```python
from build123d import *

# Parameters (mm, degrees)
SKETCH1_R               = 3.5
BOSS_EXTRUDE1_DEPTH     = 5
BOSS_EXTRUDE2_DEPTH     = 15
CHAMFER1_SIZE           = 5
CHAMFER2_SIZE           = 5
CUT_EXTRUDE1_DEPTH      = 32.721443851
CUT_EXTRUDE1_DEPTH_BACK = 32.721443851
SKETCH3_R               = 1.5
CHAMFER3_SIZE           = 2


with BuildPart() as part:
    # Sketch1 → Boss-Extrude1 (new body)
    with BuildSketch(Plane(origin=(0, 0, 0), x_dir=(1, 0, 0), z_dir=(0, 1, 0))):
        with BuildLine():
            Line((0, 6), (15.5, 6))
            ThreePointArc((15.5, 6), (21.5, 0), (15.5, -6))
            Line((15.5, -6), (-10.614590388, -6))
            Line((-10.614590388, -6), (-10.614590388, -4))
            Line((-10.614590388, -4), (0, -4))
            ThreePointArc((0, -4), (4, 0), (0, 4))
            Line((0, 4), (-10.614590388, 4))
            Line((-10.614590388, 4), (-10.614590388, 6))
            Line((-10.614590388, 6), (0, 6))
        make_face()
        with Locations(Location((15.5, 0, 0), (0, 0, 270))):
            Circle(SKETCH1_R, mode=Mode.SUBTRACT)
    extrude(amount=BOSS_EXTRUDE1_DEPTH)

    # Sketch2 → Boss-Extrude2 (add)
    with BuildSketch(Plane(origin=(0, 5, 0), x_dir=(1, 0, 0), z_dir=(0, 1, 0))):
        with BuildLine():
            Line((8.295961618, 6), (8.295961618, -6))
            Line((8.295961618, -6), (-10.614590388, -6))
            Line((-10.614590388, -6), (-10.614590388, -4))
            Line((-10.614590388, -4), (0, -4))
            ThreePointArc((0, -4), (4, 0), (0, 4))
            Line((0, 4), (-10.614590388, 4))
            Line((-10.614590388, 4), (-10.614590388, 6))
            Line((-10.614590388, 6), (8.295961618, 6))
        make_face()
    extrude(amount=BOSS_EXTRUDE2_DEPTH)

    # Chamfer1
    # the kernel refuses this chamfer: 5 mm, written as the material it takes off along each edge
    with BuildSketch(Plane(origin=(8.295961618, 20, -18.85841494), x_dir=(0.027495876610586317, -0.9996219169112968, 0), z_dir=(0, 0, 1))) as chamfer1_piece_1:
        Polygon((CHAMFER1_SIZE * 0.999621916911, -CHAMFER1_SIZE * 0.0274958766106), (-CHAMFER1_SIZE * 0.0274958766106, -CHAMFER1_SIZE * 0.999621916911), (0, 0), align=None)
    extrude(amount=37.71682988, mode=Mode.SUBTRACT)

    # Chamfer2
    chamfer2_edges = [part.edges().sort_by_distance(p)[0] for p in [
        (-10.614590388, 0, -5),
        (-10.614590388, 20, -5),
        (-10.614590388, 20, 5),
        (-10.614590388, 0, 5),
    ]]
    chamfer(chamfer2_edges, length=CHAMFER2_SIZE)

    # Sketch3 → Cut-Extrude1 (cut, two sides: drawn at the far end of the back side and taken through both)
    with BuildSketch(Plane.XY.offset(6).offset(-CUT_EXTRUDE1_DEPTH_BACK)):
        with Locations((-6.434668113, 9.88266285)):
            Circle(SKETCH3_R)
    extrude(amount=CUT_EXTRUDE1_DEPTH + CUT_EXTRUDE1_DEPTH_BACK, mode=Mode.SUBTRACT)

    # Chamfer3
    chamfer3_edges = [part.edges().sort_by_distance(p)[0] for p in [
        (8.295961618, 5, 0),
    ]]
    chamfer(chamfer3_edges, length=CHAMFER3_SIZE)


solid = part.part
```
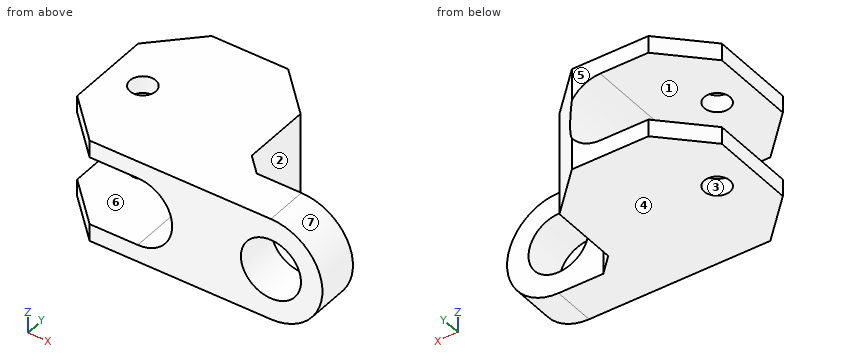
Design review of the part built by this model. Coordinates are the model's own, in mm. Face numbers are marked on the shaded views. A direction names the side the tool comes from. Coordinates: 2 decimals unless noted, no trailing zeros. Order: outer loops, then holes, each group sorted by start corner. A loop starts at its lowest first (then second) coordinate and runs counter-clockwise, first axis right, second up. Notation, with made-up numbers: M 79,58 L 99,58 A19 cw 99,70 Z; hole C 70.5,79 d2. An arc over 180 degrees is marked long. Answer as a JSON object with one key per item and string values. Group by question number.
1) Add section A-A, the plane z = 0. Write out the cut boundary in (x, y).
2) Add section D-D, the plane y = 9. Write out the cut boundary in (x, z), then the cut area to 3 significant figures.
3) Mouldability with a two-part tool opening along Z and no side actions: class the marked faces 4, 5, 6 and 7 as pulls with the +Z half, pulls with the -Z half, needs draft (parallel to the pull), parting line crosses it, or undercut.
4) Tool access review of the marked faces 1, 2 and 3: name each direction out of +Z, -Z, +X, -X, +Y, -Y from which nothing blocks a thin tool from reaching the whole face with its end or side.
5) Wall thickness on L1, parallel to Z at x = -3, y = 9; L2, parallel to X at y = 9.75, z = -5.5; L3, parallel to Y at x = 18.5, z = 4: over which ranges is each line inside the solid? List them lowest first.
6) Add section B-B, the plane y = 4.25. Write out the cut boundary in (x, z).
7) Add section C-C, the plane x = -6. Write out the cut boundary in (y, z), then the cut area to 3 significant figures.
8) For pin 1 (2.5 mm diameter, centred on x = -6.43, y = 9.88, fed in from -Z); pin 2 (1 mm diameter, centred on x = 5, z = -4.5, fed in from +Y); pin 3 (1.5 mm diameter, centred on x = 10, y = 5.5, fed in from +Z); pin 4 (4 mm diameter, centred on y = 9.5, z = -2, fed in from +X), all flat-tipped, find the tip position at first contact; note any pin that passes through.
Computed values:
{
 "1": {"outline": "M 4,0 L 12,0 L 12,5 L 10.3,5 L 8.3,7 L 8.3,15 L 4,19.3 Z; M 19,0 L 21.5,0 L 21.5,5 L 19,5 Z"},
 "2": {"outline": "M -10.61,-6 L -7.65,-6 L -7.65,-4 L -10.61,-4 Z; M -10.61,4 L -7.65,4 L -7.65,6 L -10.61,6 Z; M -5.22,-6 L 8.3,-6 L 8.3,6 L -5.22,6 L -5.22,4 L 0,4 A4 cw 0,-4 L -5.22,-4 Z", "area": "107 mm^2"},
 "3": {"face 4": "pulls with the -Z half", "face 5": "needs draft", "face 6": "undercut", "face 7": "parting line crosses it"},
 "4": {"face 1": "-X, +Y, -Y", "face 2": "+Z, -Z, +X, +Y", "face 3": "+Z, -Z"},
 "5": {"L1": "z = -6 to -4, 4 to 6", "L2": "x = -10.61 to -7.93, -4.94 to 8.3", "L3": "y = 0 to 5"},
 "6": {"outline": "M -9.86,-6 L 15.5,-6 A6 ccw 15.5,6 L -9.86,6 L -9.86,4 L 0,4 A4 cw 0,-4 L -9.86,-4 Z; hole C 15.5,0 d7"},
 "7": {"outline": "M 0.39,-6 L 8.45,-6 L 8.45,-4 L 0.39,-4 Z; M 0.39,4 L 8.45,4 L 8.45,6 L 0.39,6 Z; M 11.32,-6 L 19.61,-6 L 19.61,-4 L 11.32,-4 Z; M 11.32,4 L 19.61,4 L 19.61,6 L 11.32,6 Z", "area": "65.4 mm^2"},
 "8": {"pin 1": "passes through", "pin 2": "stops at y = 18.8", "pin 3": "stops at z = 6", "pin 4": "stops at x = 8.3"}
}
